The figure shows three views and two pictorial views of one solid part (mm, origin at its lowest corner). Answer the questions. Coordinates: 2 decimals unless noted, no trailing zeros. Write each loop counter-clockwise with the first axis right and the second up, starting at its lowest first coordinate (ties: lowest second). Pieces come first, ordered by that corner, then holes. Notation, with made-up numbers: M 77,-30.75 L 102,-30.75 A31 cw 102,-4.75 Z; hole C 80,51.5 d4. An arc over 180 degrees is marked long. Answer as CSV lines item,"result".
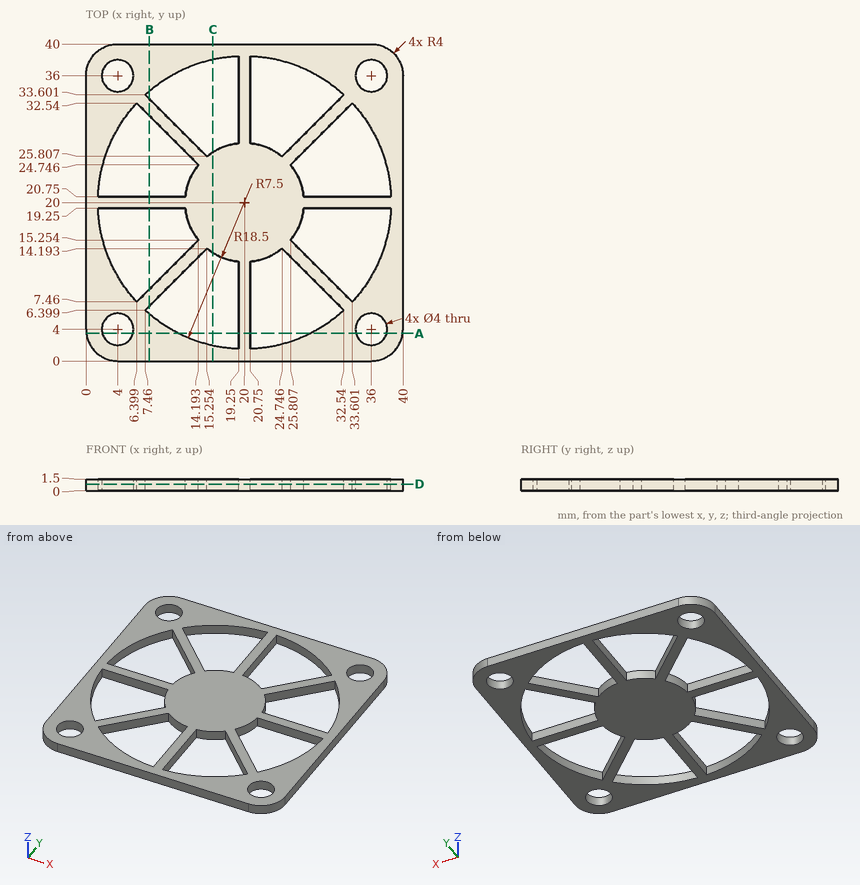
Q1. Find section C-C (x = 16). Give the vertices of the cut face in (y, z) (1 decimal).
Output:
outline,"M 0,0 L 1.9,0 L 1.9,1.5 L 0,1.5 Z; M 13.7,0 L 26.3,0 L 26.3,1.5 L 13.7,1.5 Z; M 38.1,0 L 40,0 L 40,1.5 L 38.1,1.5 Z"
Q2. Straight lines are drawn through the part: line 1 (X direction, y = 16.5, z = 1.25) (1 decimal); line 2 (X direction, y = 31.5, z = 0.2). For each, find the intervals that lie inside material, in ascending order.
Output:
line 1,"0 to 1.8, 13.4 to 26.6, 38.2 to 40"
line 2,"0 to 5.51, 7.44 to 9.56, 19.25 to 20.75, 30.44 to 32.56, 34.49 to 40"
Q3. Find section B-B (x = 8). Give the vertices of the cut face in (y, z).
Output:
outline,"M 0,0 L 5.92,0 L 5.92,1.5 L 0,1.5 Z; M 6.94,0 L 9.06,0 L 9.06,1.5 L 6.94,1.5 Z; M 19.25,0 L 20.75,0 L 20.75,1.5 L 19.25,1.5 Z; M 30.94,0 L 33.06,0 L 33.06,1.5 L 30.94,1.5 Z; M 34.08,0 L 40,0 L 40,1.5 L 34.08,1.5 Z"
Q4. Find section A-A (y = 3.5). Give the vertices of the cut face in (x, z).
Output:
outline,"M 0.03,0 L 2.06,0 L 2.06,1.5 L 0.03,1.5 Z; M 5.94,0 L 11.63,0 L 11.63,1.5 L 5.94,1.5 Z; M 19.25,0 L 20.75,0 L 20.75,1.5 L 19.25,1.5 Z; M 28.37,0 L 34.06,0 L 34.06,1.5 L 28.37,1.5 Z; M 37.94,0 L 39.97,0 L 39.97,1.5 L 37.94,1.5 Z"
Q5. Find section D-D (z = 0.85). Count the separate pieces of the cut face and the enclosed holes in it.
Output:
separate pieces,"1"
enclosed holes,"12"
